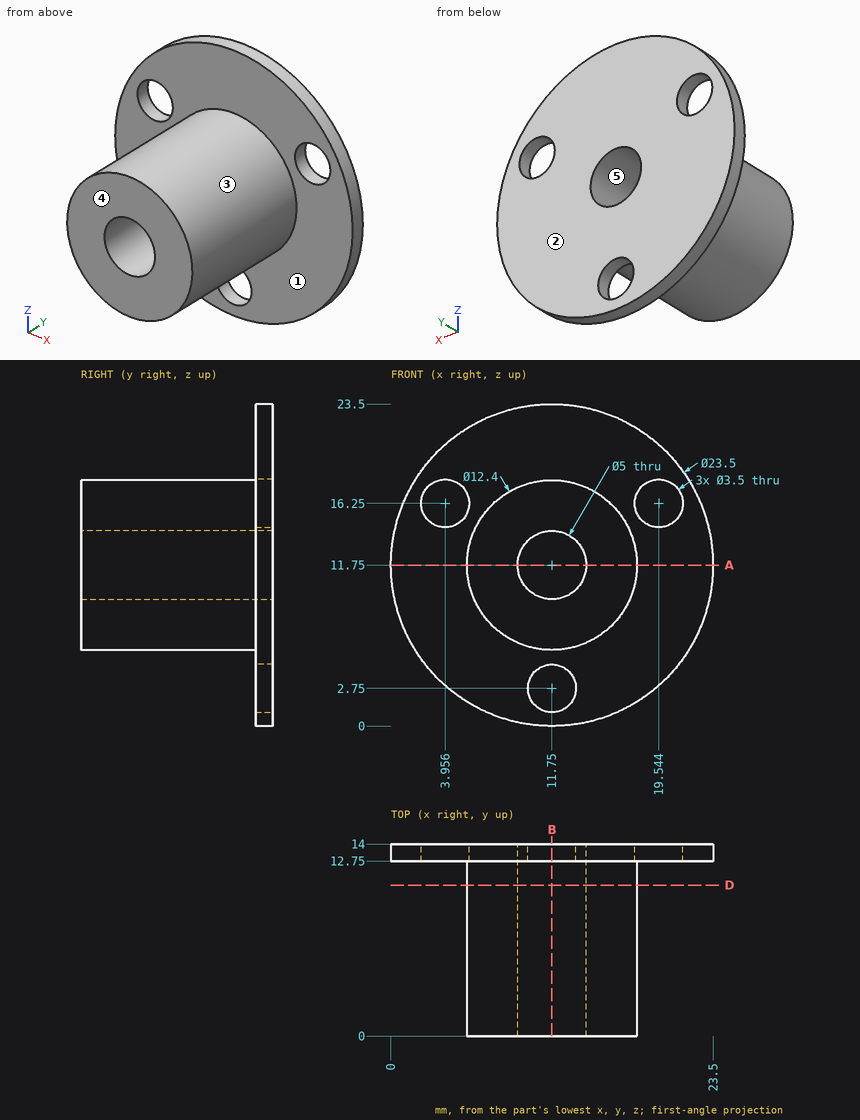
Design review of the part shown in the three views and the two pictorial views. Dimensions are in mm from the part's minimum x, y and z. A direction names the side the tool comes from. Give positions to 0.01 mm unless a question says otherwise; leave off trailing zeros. Loops run counter-clockwise (first coordinate to the right, second up) from the corner with the lowest first, then second, coordinate; pieces in that order, holes last. Notation, with made-up numbers: M -19,40 L 17,40 A6 ccw 17,50 Z; hole C 63,-15.5 d9. An arc over 180 degrees is marked long. Answer as a JSON object with one key per item and string values.
Item 1: We need section A-A (z = 11.75). State the section outline as (x, y) points.
Output values:
{"outline": "M 0,12.75 L 5.55,12.75 L 5.55,0 L 9.25,0 L 9.25,14 L 0,14 Z; M 14.25,0 L 17.95,0 L 17.95,12.75 L 23.5,12.75 L 23.5,14 L 14.25,14 Z"}
Item 2: We need section B-B (x = 11.75). State the section outline as (y, z) points.
Output values:
{"outline": "M 0,5.55 L 12.75,5.55 L 12.75,4.5 L 14,4.5 L 14,9.25 L 0,9.25 Z; M 0,14.25 L 14,14.25 L 14,23.5 L 12.75,23.5 L 12.75,17.95 L 0,17.95 Z; M 12.75,0 L 14,0 L 14,1 L 12.75,1 Z"}
Item 3: Mouldability with a two-part tool opening along Z and no side actions: class the marked faces 3, 4 and 5 as pulls with the +Z half, pulls with the -Z half, needs draft (parallel to the pull), parting line crosses it, or undercut.
Output values:
{"face 3": "parting line crosses it", "face 4": "needs draft", "face 5": "undercut"}
Item 4: Wall thickness on line 1 along Y through (x, z) = (13.75, 19.25); line 2 along X through (y, z) = (13.6, 2.75) (1 decimal); line 3 along X through (y, z) = (7.25, 13.75): over which ranges is each line inside the solid? List them lowest first.
Output values:
{"line 1": "y = 12.75 to 14", "line 2": "x = 4.2 to 10, 13.5 to 19.3", "line 3": "x = 5.88 to 10.25, 13.25 to 17.62"}
Item 5: Machinability: for the marked faces 1 and 2, which of the approach directions +Z, -Z, +X, -X, +Y, -Y give a long, thin tool a straight path to every point of the face, cutting with its end or side? Answer none if there is none.
Output values:
{"face 1": "-Y", "face 2": "+Z, -Z, +X, -X, +Y"}
Item 6: For P1, Ø6, axis at y = 7.5, z = 10, coming from the +X side; P2, Ø1.5, axis at y = 1.5, z = 6, coming from the +X side (1 decimal); P3, Ø1, axis at x = 12.5, y = 4.5, coming from the -Z side (3 decimals), all flat-tipped, find the tip position at first contact; note any pin that passes through.
Output values:
{"P1": "stops at x = 17.95", "P2": "stops at x = 15.4", "P3": "stops at z = 5.555"}
Item 7: We need section D-D (y = 11). State the section outline as (x, z) points, and give its area (3 significant figures).
Output values:
{"outline": "C 11.75,11.75 d12.4; hole C 11.75,11.75 d5", "area": "101 mm2"}
